from build123d import *

# Parameters (mm, degrees)
BOSS_EXTRUDE1_DEPTH   = 27
BOSS_EXTRUDE1_2_DEPTH = 27
BOSS_EXTRUDE2_START   = -1
BOSS_EXTRUDE2_DEPTH   = 1
BOSS_EXTRUDE3_DEPTH   = 1
SKETCH4_R             = 1
CUT_EXTRUDE1_DEPTH    = 15


with BuildPart() as part:
    # Sketch1 → Boss-Extrude1 (new body)
    with BuildSketch(Plane.XY):
        with BuildLine():
            Line((-11, 0), (-11, 22))
            ThreePointArc((-11, 22), (-8.096747752, 34.298373876), (0, 44))
            Line((0, 44), (0, 43.5))
            ThreePointArc((0, 43.5), (-7.556411695, 33.909161389), (-10.25, 22))
            Line((-10.25, 22), (-10.25, 0))
            Line((-10.25, 0), (-11, 0))
        make_face()
    extrude(amount=BOSS_EXTRUDE1_DEPTH)



with BuildPart() as body_2:
    # Sketch1 → Boss-Extrude1 2 (new body)
    with BuildSketch(Plane.XY):
        with BuildLine():
            Line((-3.5, 0), (-3.5, 22))
            ThreePointArc((-3.5, 22), (-2.616882111, 31.16856041), (0, 40))
            Line((0, 40), (0, 40.5))
            ThreePointArc((0, 40.5), (-3.173839594, 31.490949636), (-4.25, 22))
            Line((-4.25, 22), (-4.25, 0))
            Line((-4.25, 0), (-3.5, 0))
        make_face()
    extrude(amount=BOSS_EXTRUDE1_2_DEPTH)


with BuildPart() as part_1:
    add(part.part)

    add(body_2.part)  # Boss-Extrude2 merges body 2
    # Sketch2 → Boss-Extrude2 (add)
    with BuildSketch(Plane.XY.offset(27).offset(BOSS_EXTRUDE2_START)):
        with BuildLine():
            Line((-4.25, 0), (-10.25, 0))
            Line((-10.25, 0), (-10.25, 22))
            ThreePointArc((-10.25, 22), (-7.556411695, 33.909161389), (0, 43.5))
            Line((0, 43.5), (0, 40.5))
            ThreePointArc((0, 40.5), (-3.173839594, 31.490949636), (-4.25, 22))
            Line((-4.25, 22), (-4.25, 0))
        make_face()
    extrude(amount=BOSS_EXTRUDE2_DEPTH)

    # Sketch3 → Boss-Extrude3 (add)
    with BuildSketch(Plane(origin=(0, 0, 0), x_dir=(-1, 0, 0), z_dir=(0, 0, -1))):
        with BuildLine():
            Line((4.25, 0), (10.25, 0))
            Line((10.25, 0), (10.25, 22))
            ThreePointArc((10.25, 22), (7.556411695, 33.909161389), (0, 43.5))
            Line((0, 43.5), (0, 40.5))
            ThreePointArc((0, 40.5), (3.173839594, 31.490949636), (4.25, 22))
            Line((4.25, 22), (4.25, 0))
        make_face()
    extrude(amount=-BOSS_EXTRUDE3_DEPTH)

    # Sketch4 → Cut-Extrude1 (cut)
    with BuildSketch(Plane.ZY.offset(11)):
        with Locations((4.5, 2)):
            Circle(SKETCH4_R)
        with Locations((22.5, 2)):
            Circle(SKETCH4_R)
    extrude(amount=-CUT_EXTRUDE1_DEPTH, mode=Mode.SUBTRACT)


solid = part_1.part
Verification items for the finished model (mm, model axes). A direction names the side the tool comes from. Round coordinates to 2 decimals unless told otherwise and drop trailing zeros. Loops run counter-clockwise (first coordinate to the right, second up) from the corner with the lowest first, then second, coordinate; pieces in that order, holes last. Notation, with made-up numbers: (38, -30) - (62, -30) arc R32 ccw to (62, 8) - close; hole circle Ø8 at (58, 15). An arc over 180 degrees is marked (long way). Answer in a Markdown table with one row per item. Add a question column.
Q1. Section check C-C on y = 29. Enter the section's corners in (x, z).
Q2. Section check B-B on z = 6. Enter the section's corners in (x, y), plus the area to 3 significant figures.
Q3. Section check D-D on x = -7.75. Enter the section's corners in (y, z), plus the area to 3 significant figures.
Q4. Section check A-A on y = 2. Enter the section's corners in (x, z), plus the area to 3 significant figures.
Q5. Tool access check on faces 5 (the face through (-10.25, 11, 13)), 6 (the face through (-7, 17, 27)), 7 (the face through (-3.5, 11, 13)), 8 (the face through (-6, 22, 26)), 9 (the face through (-11, 11, 13)). Record the directions out of +Z, -Z, +X, -X, +Y, -Y that give a thin tool (end or side, any length) a straight path to the whole face; none if there is none.
Q6. Release check for a two-part mould opening along Y. For faces 1 (the face through (-4.25, 11, 13)), 2 (the face through (-7.482, 34.065, 13.325)), 3 (the face through (-2.64, 31.04, 13.31)), 4 (the face through (-3.144, 31.622, 13.325)) record: pulls with the +Y half, pulls with the -Y half, needs draft (parallel to the pull), parting line crosses it, or undercut.
Q7. Material ranges on line 1 (X direction, y = 17.5, z = 14.5); line 2 (Z direction, x = -8.75, y = 23), recorded low to high.
Q8. Gauge pin test, flat ends, axial feed: pin 1 (3 mm diameter, centred on y = 20.5, z = 7.5, fed in from +X); pin 2 (1 mm diameter, centred on x = -7.5, z = 14, fed in from -Y); pin 3 (1 mm diameter, centred on y = 30.5, z = 9.5, fed in from +X). Record the tip position at first contact, or that the pin passes through.
Found:
| question | item | result |
|---|---|---|
| 1 | outline | (-10.09, 0) - (-2.99, 0) - (-2.99, 27) - (-10.09, 27) - close; hole (-9.35, 1) - (-3.67, 1) - (-3.67, 26) - (-9.35, 26) - close |
| 2 | outline | (-11, 0) - (-10.25, 0) - (-10.25, 22) arc R27.67 cw to (0, 43.5) - (0, 44) arc R27.5 ccw to (-11, 22) - close; (-4.25, 0) - (-3.5, 0) - (-3.5, 22) arc R48.04 cw to (0, 40) - (0, 40.5) arc R42.39 ccw to (-4.25, 22) - close |
| 2 | area | 59.4 mm² |
| 3 | outline | (0, 0) - (34.97, 0) - (34.97, 27) - (0, 27) - (0, 26) - (33.49, 26) - (33.49, 1) - (0, 1) - close |
| 3 | area | 107 mm² |
| 4 | outline | (-11, 0) - (-3.5, 0) - (-3.5, 3.5) - (-4.25, 3.5) - (-4.25, 1) - (-10.25, 1) - (-10.25, 3.5) - (-11, 3.5) - close; (-11, 5.5) - (-10.25, 5.5) - (-10.25, 21.5) - (-11, 21.5) - close; (-11, 23.5) - (-10.25, 23.5) - (-10.25, 26) - (-4.25, 26) - (-4.25, 23.5) - (-3.5, 23.5) - (-3.5, 27) - (-11, 27) - close; (-4.25, 5.5) - (-3.5, 5.5) - (-3.5, 21.5) - (-4.25, 21.5) - close |
| 4 | area | 46.5 mm² |
| 5 | face 5 | -Y |
| 5 | face 6 | +Z, +X, -X, +Y, -Y |
| 5 | face 7 | +Z, -Z, +X, -Y |
| 5 | face 8 | none |
| 5 | face 9 | +Z, -Z, -X, +Y, -Y |
| 6 | face 1 | needs draft |
| 6 | face 2 | undercut |
| 6 | face 3 | pulls with the -Y half |
| 6 | face 4 | undercut |
| 7 | line 1 | x = -11 to -10.25, -4.25 to -3.5 |
| 7 | line 2 | z = 0 to 1, 26 to 27 |
| 8 | pin 1 | stops at x = -3.5 |
| 8 | pin 2 | stops at y = 32.93 |
| 8 | pin 3 | stops at x = -2.65 |
